The listing builds one solid part. Answer for the finished solid, in the listing's coordinates (mm). Face numbers are marked on the shaded views. A direction names the side the tool comes from. Give positions to 0.01 mm unless a question says otherwise; leave off trailing zeros. Order: outer loops, then holes, each group sorted by start corner. A loop starts at its lowest first (then second) coordinate and runs counter-clockwise, first axis right, second up.
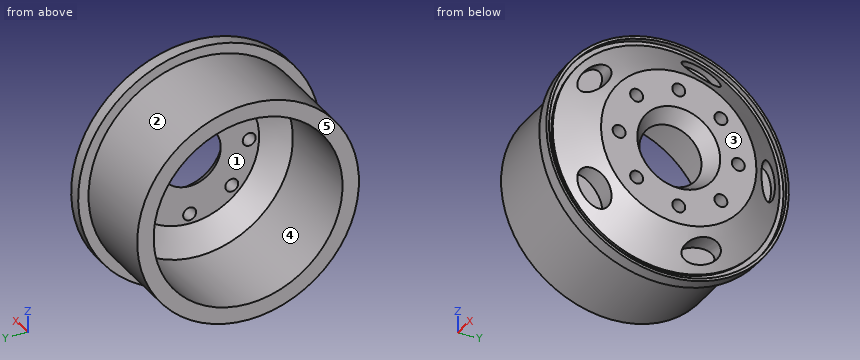
```python
from build123d import *

# Parameters (mm, degrees)
SKETCH4_R          = 1.25
SKETCH4_RX         = 4
SKETCH4_RY         = 2
CUT_EXTRUDE1_DEPTH = 5


with BuildPart() as part:
    # Sketch3 → Revolve1 (revolve)
    with BuildSketch(Plane(origin=(0, 0, 0), x_dir=(1, 0, 0), z_dir=(0, 1, 0))):
        Polygon((10.36932978, 23.4), (8.86932978, 23.4), (8.86932978, 21.4), (-8.61067022, 21.4), (-8.61067022, 18.231946605), (9.211549898, 18.231946605), (12.36932978, 13.417613419), (12.36932978, 6), (15.36932978, 8), (15.36932978, 15), (10.843535586, 21.9), (10.36932978, 21.9), (10.36932978, 22.9), (11.36932978, 22.9), (11.36932978, 23.4), align=None)
    revolve(axis=Axis((-29.774212385, 0, 0), (1, 0, 0)))

    # Sketch4 → Cut-Extrude1 (cut)
    with BuildSketch(Plane(origin=(15.36932978, 0, 0), x_dir=(0, 0, -1), z_dir=(1, 0, 0))):
        with Locations((0, 11.5)):
            Circle(SKETCH4_R)
        with Locations((8.131727984, 8.131727984)):
            Circle(SKETCH4_R)
        with Locations((11.5, 0)):
            Circle(SKETCH4_R)
        with Locations((8.131727984, -8.131727984)):
            Circle(SKETCH4_R)
        with Locations((0, -11.5)):
            Circle(SKETCH4_R)
        with Locations((-8.131727984, -8.131727984)):
            Circle(SKETCH4_R)
        with Locations((-11.5, 0)):
            Circle(SKETCH4_R)
        with Locations((-8.131727984, 8.131727984)):
            Circle(SKETCH4_R)
        with Locations((0, 18.5)):
            Ellipse(SKETCH4_RX, SKETCH4_RY)
        with Locations(Location((17.594545551, 5.716814396), (0, 0, -72))):
            Ellipse(SKETCH4_RX, SKETCH4_RY)
        with Locations(Location((10.874027167, -14.966814396), (0, 0, -144))):
            Ellipse(SKETCH4_RX, SKETCH4_RY)
        with Locations(Location((-10.874027167, -14.966814396), (0, 0, 144))):
            Ellipse(SKETCH4_RX, SKETCH4_RY)
        with Locations(Location((-17.594545551, 5.716814396), (0, 0, 72))):
            Ellipse(SKETCH4_RX, SKETCH4_RY)
    extrude(amount=-CUT_EXTRUDE1_DEPTH, mode=Mode.SUBTRACT)


solid = part.part
```
1) For a pull along Z with two mould halves and no side action, classify the marked faces 1, 2 and 3 as +Z half, -Z half, draft (parallel to the pull), parting line (faces both ways), or undercut.
Geometry says:
face 1: undercut
face 2: parting line
face 3: draft
2) Given P1, Ø6, axis at x = 6, z = -5, coming from the +Y side; P2, Ø2, axis at y = -11.5, z = 0, coming from the +X side; P3, Ø21.5, axis at y = 2.5, z = -5, coming from the -X side; P4, Ø4, axis at x = -4, z = 0, coming from the +Y side, each flat-ended and moving along its own axis, determine where each tip first touches the part or whether it passes through.
Geometry says:
P1: stops at y = 23.03
P2: passes through
P3: stops at x = 10.45
P4: stops at y = 21.4
3) Find section B-B (x = 5). Write down the section's boundary in (y, z).
Geometry says:
outline: circle Ø42.8 at (0, 0); hole circle Ø36.46 at (0, 0)
4) Straight lines are drawn through the part: probe 1 along Y at (x, z) = (14.05, 0); probe 2 along Y at (x, z) = (13.3, 0); probe 3 along Y at (x, z) = (-6, -2). For each, find the intervals that lie inside material, in ascending order.
Geometry says:
probe 1: y = -17.01 to -12.75, -10.25 to -7.12, 7.12 to 10.25, 12.75 to 16.5
probe 2: y = -18.15 to -12.75, -10.25 to -6.62, 6.62 to 10.25, 12.75 to 16.5
probe 3: y = -21.31 to -18.12, 18.12 to 21.31
5) Find section A-A (y = 0). Count the separate pieces of the cut face and the enclosed holes in it, then the cut area to 3 significant figures.
Geometry says:
separate pieces: 4
enclosed holes: 0
area: 200 mm2
6) A tool of negligible diameter and unlimited length cuts with its end or side. For the marked faces 4 and 5, from which of +Z, -Z, +X, -X, +Y, -Y can it reach the whole face along a straight path? Write none if from no direction.
Geometry says:
face 4: -X
face 5: +Z, -Z, -X, +Y, -Y
